from build123d import *

# Parameters (mm, degrees)
MAIN_BLOCK_DEPTH    = 4
M5_TAPPED_SECTION_D = 4.2
COSMETIC_FILLETS_R  = 0.4


with BuildPart() as part:
    # Main Block Sketch → Main Block (new body)
    with BuildSketch(Plane(origin=(0, 0, 0), x_dir=(1, 0, 0), z_dir=(0, 1, 0))):
        Polygon((2.309401077, 4), (-2.309401077, 4), (-4.618802154, 0), (-2.309401077, -4), (2.309401077, -4), (4.618802154, 0), align=None)
    extrude(amount=MAIN_BLOCK_DEPTH)

    # M5 Tapped section (through all)
    with Locations(Plane(origin=(0, 0, 0), x_dir=(-1, 0, 0), z_dir=(0, -1, 0))):
        with Locations((0, 0)):
            Hole(M5_TAPPED_SECTION_D / 2)

    # Cosmetic Fillets
    cosmetic_fillets_edges = [part.edges().sort_by_distance(p)[0] for p in [
        (4.618802154, 2, 0),
        (2.309401077, 2, 4),
        (-2.309401077, 2, 4),
        (-4.618802154, 2, 0),
        (-2.309401077, 2, -4),
        (2.309401077, 2, -4),
        (-3.464101615, 4, -2),
        (-3.464101615, 4, 2),
        (0, 4, 4),
        (-2.1, 0, 0),
        (-2.1, 4, 0),
        (3.464101615, 4, 2),
        (3.464101615, 4, -2),
        (3.464101615, 0, 2),
        (0, 0, 4),
        (-3.464101615, 0, 2),
        (-3.464101615, 0, -2),
        (0, 0, -4),
        (3.464101615, 0, -2),
        (0, 4, -4),
    ]]
    fillet(cosmetic_fillets_edges, radius=COSMETIC_FILLETS_R)


solid = part.part
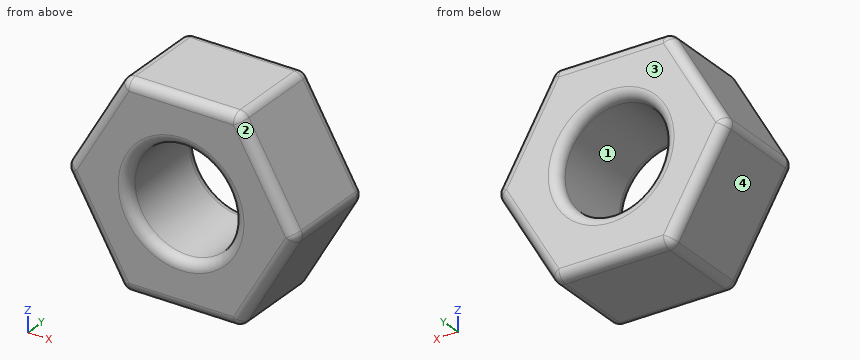
Here's how the part is built. I have some questions about the finished solid (model axes, mm). Face numbers are marked on the shaded views. Round coordinates to 2 decimals unless told otherwise and drop trailing zeros. Loops run counter-clockwise (first coordinate to the right, second up) from the corner with the lowest first, then second, coordinate; pieces in that order, holes last. Notation, with made-up numbers: (5.5, 51.5) - (44.5, 51.5) arc R19 ccw to (44.5, 73.5) - close; hole circle Ø4 at (85, 44.25). An arc over 180 degrees is marked (long way). One line per question, with ' | ' between items. Start each with the question number.
Q1. We'd pull the mould along Z, two halves only. Please class the marked faces 1, 2, 3 and 4: +Z half, -Z half, draft (parallel to the pull), parting line (faces both ways), or undercut.
Q2. Will these pins go through, and if not, where does the flat tip stop? pin 1 (4 mm diameter, centred on x = -1.5, z = -2.5, fed in from -Y); pin 2 (1 mm diameter, centred on y = 1.5, z = -1.5, fed in from -X); pin 3 (1.5 mm diameter, centred on y = 1.5, z = -1.5, fed in from -X).
Q3. I want a section at A-A (x = 0). Write out the boundary of the cut face in (y, z).
Q4. I want a section at B-B (y = 1.7). Write out the boundary of the cut face in (x, z), then the cut area to 3 significant figures.
Q5. Please list where these lines run through material, in increasing order: line 1 (Z direction, x = 0, y = 0.75); line 2 (X direction, y = 2.95, z = 0); line 3 (X direction, y = 2.1, z = -0.5). Write a range as [from, to].
Response values:
1) face 1: undercut | face 2: +Z half | face 3: draft | face 4: -Z half
2) pin 1: stops at y = 0 | pin 2: stops at x = -4.04 | pin 3: stops at x = -4.19
3) outline: (0, -3.6) arc R0.4 ccw to (0.4, -4) - (3.6, -4) arc R0.4 ccw to (4, -3.6) - (4, -2.5) arc R0.4 ccw to (3.6, -2.1) - (0.4, -2.1) arc R0.4 ccw to (0, -2.5) - close; (0, 2.5) arc R0.4 ccw to (0.4, 2.1) - (3.6, 2.1) arc R0.4 ccw to (4, 2.5) - (4, 3.6) arc R0.4 ccw to (3.6, 4) - (0.4, 4) arc R0.4 ccw to (0, 3.6) - close
4) outline: (-4.5, -0.2) - (-2.42, -3.8) arc R0.4 ccw to (-2.08, -4) - (2.08, -4) arc R0.4 ccw to (2.42, -3.8) - (4.5, -0.2) arc R0.4 ccw to (4.5, 0.2) - (2.42, 3.8) arc R0.4 ccw to (2.08, 4) - (-2.08, 4) arc R0.4 ccw to (-2.42, 3.8) - (-4.5, 0.2) arc R0.4 ccw to start; hole circle Ø4.2 at (0, 0) | area: 41.5 mm²
5) line 1: z = [-4, -2.1], [2.1, 4] | line 2: x = [-4.56, -2.1], [2.1, 4.56] | line 3: x = [-4.33, -2.04], [2.04, 4.33]
